```python
from build123d import *

# Parameters (mm, degrees)
SKETCH1_W           = 27
SKETCH1_H           = 29
BOSS_EXTRUDE1_DEPTH = 5
SKETCH3_R           = 1.1
CUT_EXTRUDE2_DEPTH  = 10
SKETCH4_W           = 21
SKETCH4_H           = 8.5
CUT_EXTRUDE3_DEPTH  = 10
SKETCH2_R           = 1.2
BOSS_EXTRUDE2_DEPTH = 2
SKETCH7_W           = 3
SKETCH7_H           = 3
BOSS_EXTRUDE5_DEPTH = 1.5
SKETCH8_W           = 27
SKETCH8_H           = 0.75
BOSS_EXTRUDE6_DEPTH = 4


with BuildPart() as part:
    # Sketch1 → Boss-Extrude1 (new body)
    with BuildSketch(Plane.XY):
        Rectangle(SKETCH1_W, SKETCH1_H)
    extrude(amount=BOSS_EXTRUDE1_DEPTH)

    # Sketch3 → Cut-Extrude2 (cut)
    with BuildSketch(Plane.XY.offset(5)):
        with Locations((-10.7, 12.7)):
            Circle(SKETCH3_R)
        with Locations((10.5, 12.7)):
            Circle(SKETCH3_R)
        with Locations((-10.7, 3.025)):
            Circle(SKETCH3_R)
        with Locations((10.5, 3.025)):
            Circle(SKETCH3_R)
    extrude(amount=-CUT_EXTRUDE2_DEPTH, mode=Mode.SUBTRACT)

    # Sketch4 → Cut-Extrude3 (cut)
    with BuildSketch(Plane.XY.offset(5)):
        with Locations((0, -7.429078055)):
            Rectangle(SKETCH4_W, SKETCH4_H)
    extrude(amount=-CUT_EXTRUDE3_DEPTH, mode=Mode.SUBTRACT)

    # Sketch2 → Boss-Extrude2 (add)
    with BuildSketch(Plane.XZ.offset(14.5)):
        with Locations(Location((-7, 2.5, 0), (0, 0, 90))):
            Circle(SKETCH2_R)
        with Locations(Location((0, 2.5, 0), (0, 0, 90))):
            Circle(SKETCH2_R)
        with Locations(Location((7, 2.5, 0), (0, 0, 90))):
            Circle(SKETCH2_R)
    extrude(amount=BOSS_EXTRUDE2_DEPTH)

    # Sketch7 → Boss-Extrude5 (add)
    with BuildSketch(Plane(origin=(0, 0, 0), x_dir=(-1, 0, 0), z_dir=(0, 0, -1))):
        with Locations((-12, -4.679078055)):
            Rectangle(SKETCH7_W, SKETCH7_H)
        with Locations((12, -4.679078055)):
            Rectangle(SKETCH7_W, SKETCH7_H)
    extrude(amount=BOSS_EXTRUDE5_DEPTH)

    # Sketch8 → Boss-Extrude6 (add)
    with BuildSketch(Plane(origin=(0, -3.179078055, 0), x_dir=(1, 0, 0), z_dir=(0, 1, 0))):
        with Locations((0, 1.125)):
            Rectangle(SKETCH8_W, SKETCH8_H)
    extrude(amount=BOSS_EXTRUDE6_DEPTH)


solid = part.part
```
For this review, take the finished solid that the model builds, in its own axes (mm). A direction names the side the tool comes from. Round coordinates to 2 decimals unless told otherwise and drop trailing zeros. Write each loop counter-clockwise with the first axis right and the second up, starting at its lowest first coordinate (ties: lowest second). Pieces come first, ordered by that corner, then holes.
1) For line 1 along X through (y, z) = (3, 0.75); line 2 along X through (y, z) = (-10, 1); line 3 along Z through (x, y) = (-5.5, 0), list the stretches that pass through material, from the lowest coordinate up.
Answer below:
line 1: x = -13.5 to -11.8, -9.6 to 9.4, 11.6 to 13.5
line 2: x = -13.5 to -10.5, 10.5 to 13.5
line 3: z = -1.5 to -0.75, 0 to 5
2) Machinability: for faces 1 (the face through (-0.36, -15.486, 3.645)), 2 (the face through (12, -6.179, -1)), 3 (the face through (0, -2, -1.5)), 4 (the face through (10.5, -7, 3)), which of the approach directions +Z, -Z, +X, -X, +Y, -Y give a long, thin tool a straight path to every point of the face, cutting with its end or side? Answer none if there is none.
Answer below:
face 1: -Y
face 2: -Z, +X, -X, -Y
face 3: -Z, +X, -X, +Y, -Y
face 4: +Z, -Z
3) Take a section at B-B on x = -2.75. Give the boundary of the cut face in (y, z), then the cut area to 4 significant figures.
Answer below:
outline: (-14.5, 0) - (-11.68, 0) - (-11.68, 5) - (-14.5, 5) - close; (-3.18, -1.5) - (0.82, -1.5) - (0.82, -0.75) - (-3.18, -0.75) - close; (-3.18, 0) - (14.5, 0) - (14.5, 5) - (-3.18, 5) - close
area: 105.5 mm2
4) Take a section at C-C on y = -2. Give the boundary of the cut face in (x, z).
Answer below:
outline: (-13.5, -1.5) - (13.5, -1.5) - (13.5, -0.75) - (-13.5, -0.75) - close; (-13.5, 0) - (13.5, 0) - (13.5, 5) - (-13.5, 5) - close
5) Insertion check: pin 1 Ø4 at (x, y) = (-6.5, -11) entering from -Z; pin 2 Ø2 at (x, z) = (0, -0.5) entering from +Y; pin 3 Ø0.8 at (x, z) = (-12.5, -0.5) entering from +Y; pin 4 Ø1.6 at (x, z) = (11.5, -1) entering from -Y. Each pin has a flat end and moves straight along its axis. Give the tip position at first contact, or say it passes through.
Answer below:
pin 1: stops at z = 0
pin 2: stops at y = 14.5
pin 3: stops at y = 0.82
pin 4: stops at y = -6.18
6) Take a section at D-D on z = 2.25. Give the boundary of the cut face in (x, y) (3 decimals), then the cut area to 3 significant figures.
Answer below:
outline: (-13.5, -14.5) - (-8.174, -14.5) - (-8.174, -16.5) - (-5.826, -16.5) - (-5.826, -14.5) - (-1.174, -14.5) - (-1.174, -16.5) - (1.174, -16.5) - (1.174, -14.5) - (5.826, -14.5) - (5.826, -16.5) - (8.174, -16.5) - (8.174, -14.5) - (13.5, -14.5) - (13.5, 14.5) - (-13.5, 14.5) - close; hole circle Ø2.2 at (-10.7, 3.025); hole circle Ø2.2 at (-10.7, 12.7); hole (-10.5, -11.679) - (10.5, -11.679) - (10.5, -3.179) - (-10.5, -3.179) - close; hole circle Ø2.2 at (10.5, 3.025); hole circle Ø2.2 at (10.5, 12.7)
area: 603 mm2
7) Mouldability with a two-part tool opening along Z and no side actions: class faces 5 (the face through (13.5, 0, 3)), 6 (the face through (0, 3, 5)), 7 (the face through (0, -1, -0.75)) as +Z half, -Z half, draft (parallel to the pull), parting line (faces both ways), or undercut.
Answer below:
face 5: draft
face 6: +Z half
face 7: undercut
8) Take a section at A-A on y = 12.7. Give the boundary of the cut face in (x, z).
Answer below:
outline: (-13.5, 0) - (-11.8, 0) - (-11.8, 5) - (-13.5, 5) - close; (-9.6, 0) - (9.4, 0) - (9.4, 5) - (-9.6, 5) - close; (11.6, 0) - (13.5, 0) - (13.5, 5) - (11.6, 5) - close
